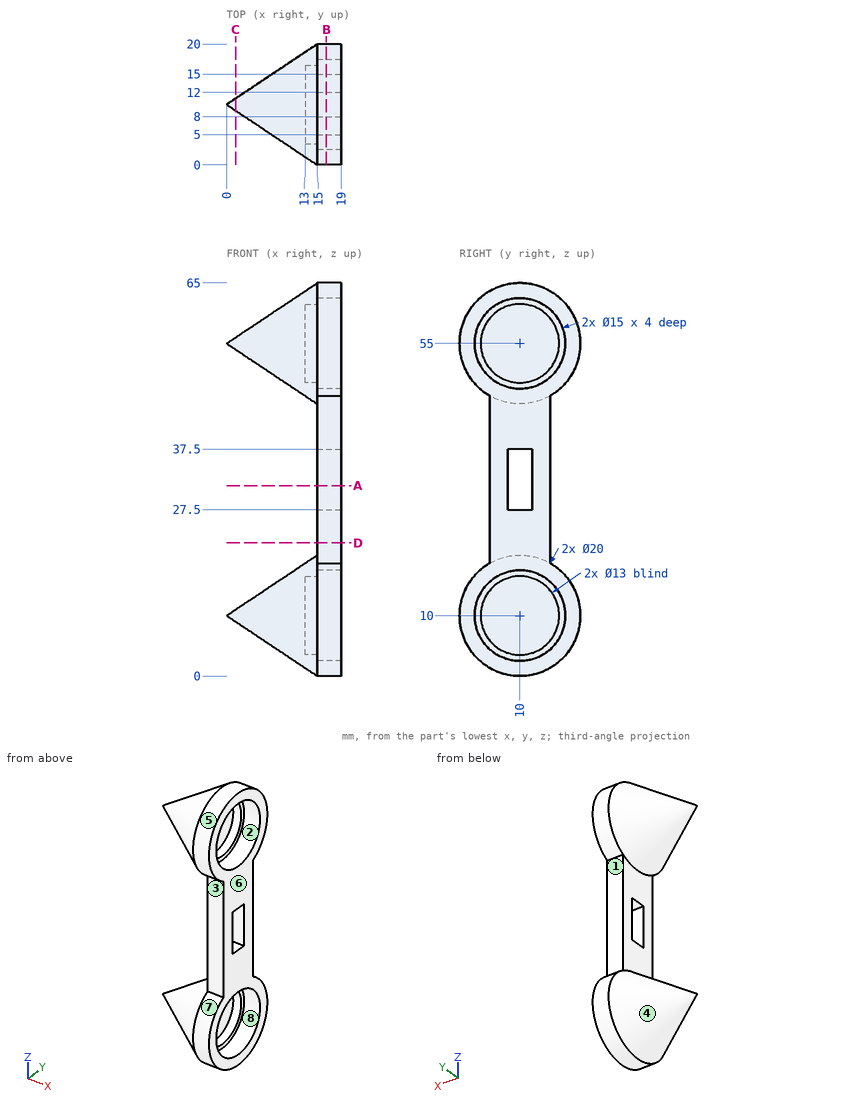
Part print with two shaded views. Sizes in mm from the minimum x, y, z corner. A direction names the side the tool comes from. Coordinates: 2 decimals unless noted, no trailing zeros. Write each loop counter-clockwise with the first axis right and the second up, starting at its lowest first coordinate (ties: lowest second). Pieces come first, ordered by that corner, then holes.
(1) Drill centre lines: line 1 (Z direction, x = 16.5, y = 10); line 2 (Y direction, x = 17.7, z = 55); line 3 (Z direction, x = 12.25, y = 4.25). Where is each one in solid material? Low to high.
(2) Mould opens along Y. For the marked faces 6, 7 and 8 say: pulls with the +Y half, pulls with the -Y half, needs draft (parallel to the pull), parting line crosses it, or undercut.
(3) Cut at D-D on z = 22. List the corners of the cut face in (x, y), and give its area (3 significant figures).
(4) Cut at A-A on z = 31.5. List the corners of the cut face in (x, y).
(5) Cut at C-C on x = 1.5. List the corners of the cut face in (y, z), and give its area (3 significant figures).
(6) 3-axis set-ups, long thin cutter, end or side, ignore diameter. For the marked faces 1, 2, 3, 4 and 5: which of +Z, -Z, +X, -X, +Y, -Y reach the whole face in a straight line?
(7) Pin check, flat tips, straight feed: pin 1 Ø8 at (y, z) = (13, 42) entering from -X; pin 2 Ø2 at (y, z) = (7.5, 56.5) entering from +X; pin 3 Ø1.2 at (x, z) = (18, 32.5) entering from +Y; pin 4 Ø8 at (x, y) = (12.5, 10) entering from -Z. Stop position of each tip, or through.
(8) Cut at B-B on x = 16.5. List the corners of the cut face in (y, z).
Working result:
1. line 1: z = 0 to 2.5, 17.5 to 27.5, 37.5 to 47.5, 62.5 to 65
1. line 2: y = 0 to 2.5, 17.5 to 20
1. line 3: z = 4.2 to 15.8, 49.2 to 60.8
2. face 6: needs draft
2. face 7: parting line crosses it
2. face 8: undercut
3. outline: (15, 5) - (19, 5) - (19, 15) - (15, 15) - close
3. area: 40.0 mm2
4. outline: (15, 5) - (19, 5) - (19, 8) - (15, 8) - close; (15, 12) - (19, 12) - (19, 15) - (15, 15) - close
5. outline: circle Ø2 at (10, 10); circle Ø2 at (10, 55)
5. area: 6.28 mm2
6. face 1: +X, -X, +Y
6. face 2: +X
6. face 3: +X, -X, -Y
6. face 4: -X
6. face 5: +X, -X
7. pin 1: stops at x = 14.01
7. pin 2: stops at x = 13
7. pin 3: stops at y = 15
7. pin 4: stops at z = 0
8. outline: (5, 18.66) arc R10 ccw (long way) to (15, 18.66) - (15, 46.34) arc R10 ccw (long way) to (5, 46.34) - close; hole circle Ø15 at (10, 10); hole circle Ø15 at (10, 55); hole (8, 27.5) - (12, 27.5) - (12, 37.5) - (8, 37.5) - close
